For this review, use the dimensioned drawing (mm, ordinates from the lowest corner) and the shaded views. A direction names the side the tool comes from. Round coordinates to 2 decimals unless told otherwise and drop trailing zeros. Order: outer loops, then holes, each group sorted by start corner. A loop starts at its lowest first (then second) coordinate and runs counter-clockwise, first axis right, second up. Notation, with made-up numbers: M 11.25,-35 L 23.25,-35 A34 cw 23.25,-2 Z; hole C -24.5,14.25 d3. An arc over 180 degrees is marked long. Use a Markdown table: item, result. Add a question column.
1. Consider section B-B on x = 40. State the section outline as (y, z) points, then the cut area to 3 significant figures.
2. For the marked faces 4 and 5, list the 3-axis set-ups (+Z, -Z, +X, -X, +Y, -Y) from which the entire face can be reached by the end or side of a thin tool; tool diameter is ignored.
3. To check wall thickness, follow probe 1 along Y at (x, z) = (160, 9.75); probe 2 along Y at (x, z) = (40, 30.25); probe 3 along Z at (x, y) = (163.5, 104.5). State the ranges of each line that lie inside material, in increasing order.
4. Consider section C-C on y = 40. State the section outline as (x, z) points, then the cut area to 3 significant figures.
5. Insertion check: P1, Ø20, axis at x = 40, y = 160, coming from the +Z side; P2, Ø16, axis at x = 34.5, y = 166, coming from the +Z side; P3, Ø18, axis at x = 234.5, z = 80.5, coming from the +Y side. Each pin has a flat end and moves straight along its axis. Give the tip position at first contact, or say it passes through.
6. Consider section A-A on y = 100. State the section outline as (x, z) points.
7. The part is to be moulded in two halves that separate along Z. For the marked faces 1, 2 and 3, say which applies: +Z half, -Z half, draft (parallel to the pull), parting line (faces both ways), or undercut.
8. Consider section D-D on z = 75.5. State the section outline as (x, y) points.
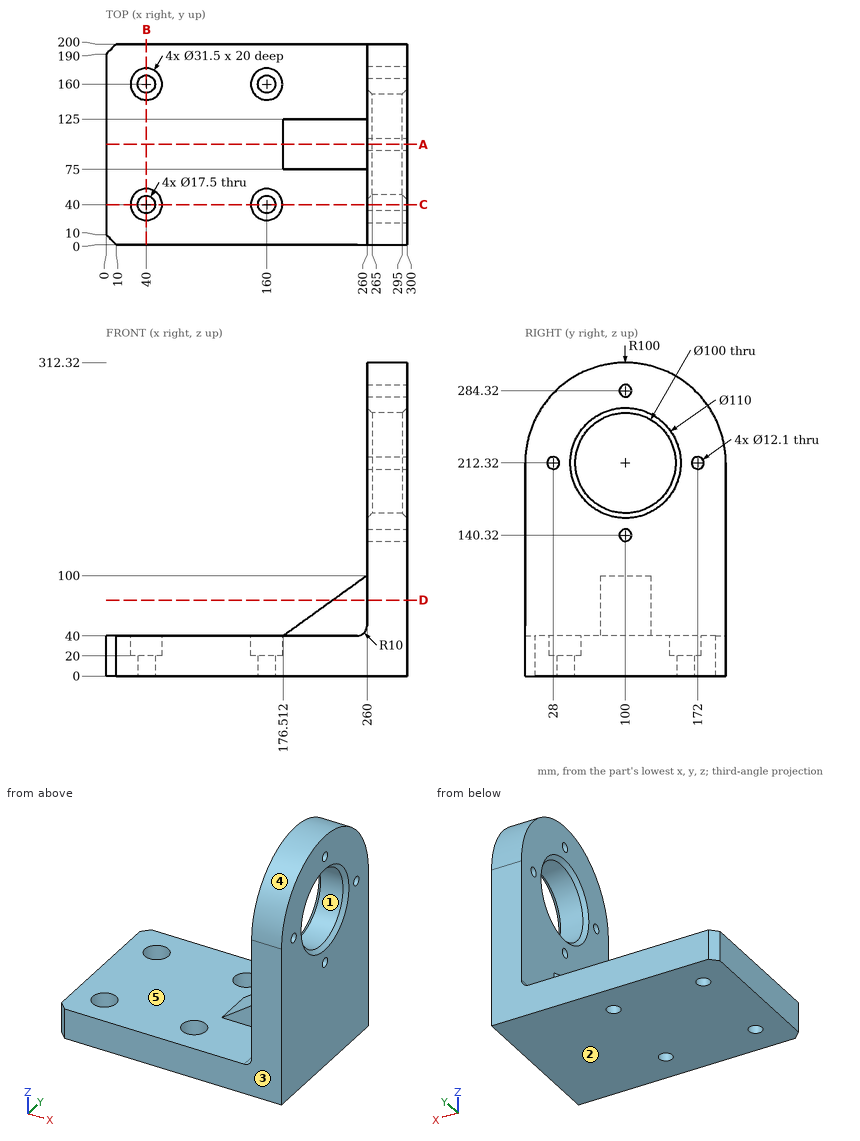
Answer block:
| question | item | result |
|---|---|---|
| 1 | outline | M 0,0 L 31.25,0 L 31.25,20 L 24.25,20 L 24.25,40 L 0,40 Z; M 48.75,0 L 151.25,0 L 151.25,20 L 144.25,20 L 144.25,40 L 55.75,40 L 55.75,20 L 48.75,20 Z; M 168.75,0 L 200,0 L 200,40 L 175.75,40 L 175.75,20 L 168.75,20 Z |
| 1 | area | 6,040 mm^2 |
| 2 | face 4 | +Z, +X, -X |
| 2 | face 5 | +Z, -X |
| 3 | probe 1 | 0 to 31.25, 48.75 to 151.25, 168.75 to 200 |
| 3 | probe 2 | 0 to 24.25, 55.75 to 144.25, 175.75 to 200 |
| 3 | probe 3 | 0 to 40 |
| 4 | outline | M 0,0 L 31.25,0 L 31.25,20 L 24.25,20 L 24.25,40 L 0,40 Z; M 48.75,0 L 151.25,0 L 151.25,20 L 144.25,20 L 144.25,40 L 55.75,40 L 55.75,20 L 48.75,20 Z; M 168.75,0 L 300,0 L 300,292.32 L 260,292.32 L 260,50 A10 cw 250,40 L 175.75,40 L 175.75,20 L 168.75,20 Z |
| 4 | area | 20,200 mm^2 |
| 5 | P1 | z = 20 |
| 5 | P2 | z = 40 |
| 5 | P3 | y = 125 |
| 6 | outline | M 0,0 L 300,0 L 300,134.27 L 260,134.27 L 260,100 L 176.51,40 L 0,40 Z; M 260,146.37 L 300,146.37 L 300,157.32 L 295,162.32 L 265,162.32 L 260,157.32 Z; M 260,267.32 L 265,262.32 L 295,262.32 L 300,267.32 L 300,278.27 L 260,278.27 Z; M 260,290.37 L 300,290.37 L 300,312.32 L 260,312.32 Z |
| 7 | face 1 | undercut |
| 7 | face 2 | -Z half |
| 7 | face 3 | draft |
| 8 | outline | M 225.91,75 L 260,75 L 260,0 L 300,0 L 300,200 L 260,200 L 260,125 L 225.91,125 Z |
